Geometry check sheet. Reference: drawing and pictorial views, mm from the part's lowest x, y, z. A direction names the side the tool comes from. Coordinates: 2 decimals unless noted, no trailing zeros. Loops run counter-clockwise (first coordinate to the right, second up) from the corner with the lowest first, then second, coordinate; pieces in that order, holes last. Notation, with made-up numbers: (68.5, 8.25) -> (79.5, 8.25) arc R24 ccw to (79.5, 33.25) -> close; hole circle Ø7 at (72, 59). An arc over 180 degrees is marked (long way). Use CSV: the item, a comma, the result in double quotes.
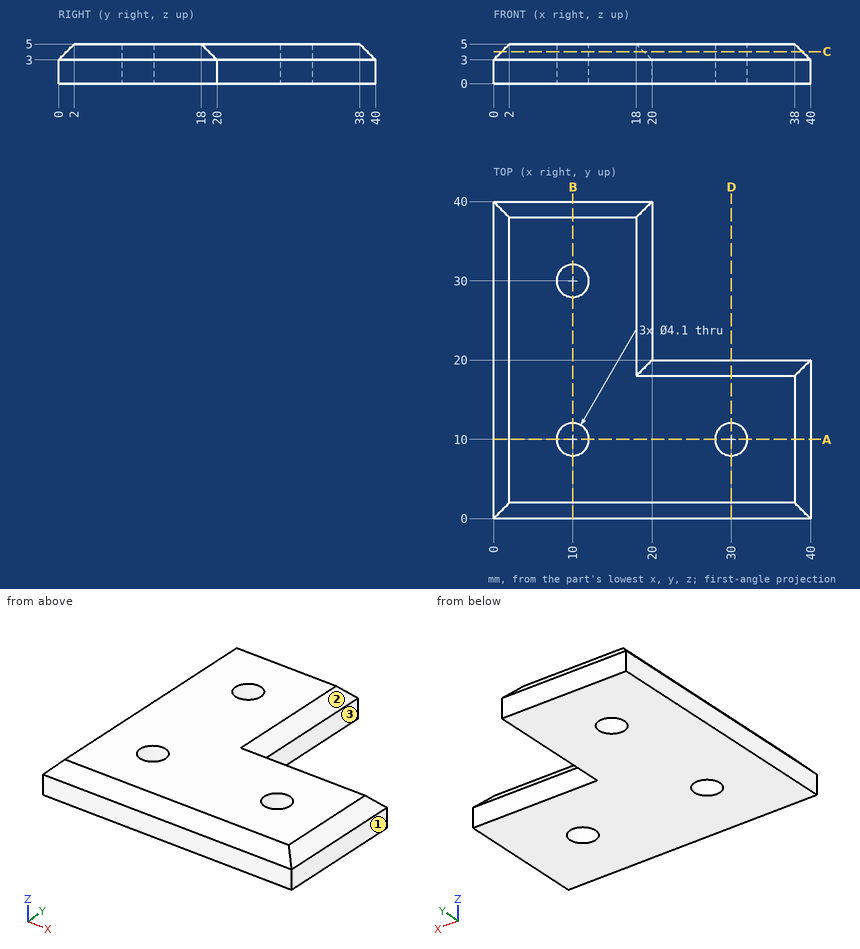
1) Cross-section at D-D on x = 30. Record the boundary of the cut face in (y, z).
Answer below:
outline,"(0, 0) -> (7.95, 0) -> (7.95, 5) -> (2, 5) -> (0, 3) -> close; (12.05, 0) -> (20, 0) -> (20, 3) -> (18, 5) -> (12.05, 5) -> close"
2) Go/stop test with flat-tipped pins: pin 1 Ø3.5 at (x, y) = (10, 30) entering from -Z; pin 2 Ø1.5 at (x, z) = (34, 1) entering from +Y; pin 3 Ø1.5 at (y, z) = (28, 1) entering from +X. Record where each tip stops, or that it passes through.
Answer below:
pin 1,"passes through"
pin 2,"stops at y = 20"
pin 3,"stops at x = 20"
3) Cross-section at C-C on z = 4.05. Record the boundary of the cut face in (x, y), and give its area (3 significant figures).
Answer below:
outline,"(1.05, 1.05) -> (38.95, 1.05) -> (38.95, 18.95) -> (18.95, 18.95) -> (18.95, 38.95) -> (1.05, 38.95) -> close; hole circle Ø4.1 at (10, 10); hole circle Ø4.1 at (10, 30); hole circle Ø4.1 at (30, 10)"
area,"997 mm²"
4) Cross-section at A-A on y = 10. Record the boundary of the cut face in (x, z), and give its area (3 significant figures).
Answer below:
outline,"(0, 0) -> (7.95, 0) -> (7.95, 5) -> (2, 5) -> (0, 3) -> close; (12.05, 0) -> (27.95, 0) -> (27.95, 5) -> (12.05, 5) -> close; (32.05, 0) -> (40, 0) -> (40, 3) -> (38, 5) -> (32.05, 5) -> close"
area,"155 mm²"
5) Access from +Z, -Z, +X, -X, +Y, -Y to the whole of each face (thin tool, end or side, straight path). Record for the marked faces 1, 2 and 3.
Answer below:
face 1,"+Z, -Z, +X, +Y, -Y"
face 2,"+Z, +X, +Y"
face 3,"+Z, -Z, +X, +Y"
6) Thickness scan on line 1 along Y through (x, z) = (10, 1); line 2 along X through (y, z) = (8.5, 4.1); line 3 along Y through (x, z) = (10, 3.6). Record the ranges inside material, lowest first. Write a range as from..to.
Answer below:
line 1,"y = 0..7.95, 12.05..27.95, 32.05..40"
line 2,"x = 1.1..8.6, 11.4..28.6, 31.4..38.9"
line 3,"y = 0.6..7.95, 12.05..27.95, 32.05..39.4"
